Design review of the part built by this model. Coordinates are the model's own, in mm. A direction names the side the tool comes from. Round coordinates to 2 decimals unless told otherwise and drop trailing zeros. Loops run counter-clockwise (first coordinate to the right, second up) from the corner with the lowest first, then second, coordinate; pieces in that order, holes last. Notation, with made-up numbers: M -9.5,69.5 L 42.5,69.5 A21 ccw 42.5,77.5 Z; hole C 41.5,29.25 d8. An arc over 180 degrees is marked long. Use a Markdown table: item, result.
from build123d import *

# Parameters (mm, degrees)
SKETCH_W            = 120.815
SKETCH_H            = 65.873
PAD_DEPTH           = 25
POCKET_DEPTH        = 17
SKETCH002_R         = 0.8
HOLE_DEPTH          = 8.001
SKETCH003_W         = 10.80455
SKETCH003_H         = 10.011545
SKETCH003_W_2       = 3
SKETCH003_H_2       = 20
SKETCH003_W_3       = 21
SKETCH003_H_3       = 14
SKETCH003_W_4       = 17.5
SKETCH003_H_4       = 8
SKETCH003_W_5       = 4
SKETCH003_H_5       = 15
SKETCH003_W_6       = 39.832252
SKETCH003_H_6       = 6.416744
PAD001_DEPTH        = 14
HOLE001_D           = 3.5
HOLE001_DEPTH       = 20
HOLE001_CBORE_D     = 4.2
HOLE001_CBORE_DEPTH = 5
POCKET001_DEPTH     = 120.816


with BuildPart() as part:
    # Sketch → Pad (new body)
    with BuildSketch(Plane.XY):
        with Locations((50.4075, 22.9365)):
            Rectangle(SKETCH_W, SKETCH_H)
    extrude(amount=-PAD_DEPTH)

    # Sketch001 (on Face5 of Pad) → Pocket (cut)
    with BuildSketch(Plane.XY):
        Polygon((-0.5, 40.5), (-0.5, -0.5), (17.5, -0.5), (17.5, 5.25), (40.721178, 5.25), (40.721178, -0.5), (101.315, -0.5), (101.315, 40.5), (96.315, 40.5), (96.315, 50.5), (9.5, 50.5), (9.5, 40.5), align=None)
    extrude(amount=-POCKET_DEPTH, mode=Mode.SUBTRACT)

    # Sketch002 (on Face19 of Pocket) → Hole (cut, through all)
    with BuildSketch(Plane.XY.offset(-17)):
        with Locations((60.8, 35.99)):
            Circle(SKETCH002_R)
        with Locations((63.34, 35.99)):
            Circle(SKETCH002_R)
        with Locations((65.88, 35.99)):
            Circle(SKETCH002_R)
        with Locations((65.88, 33.45)):
            Circle(SKETCH002_R)
        with Locations((63.34, 33.45)):
            Circle(SKETCH002_R)
        with Locations((60.8, 33.45)):
            Circle(SKETCH002_R)
    extrude(amount=-HOLE_DEPTH, mode=Mode.SUBTRACT)

    # Sketch003 (on Face25 of Hole) → Pad001 (join)
    with BuildSketch(Plane.XY.offset(-17)):
        with Locations((82.816269, 15.264502)):
            Rectangle(SKETCH003_W, SKETCH003_H)
        with Locations((99.815, 30.5)):
            Rectangle(SKETCH003_W_2, SKETCH003_H_2)
        with Locations((51.221178, 6.5)):
            Rectangle(SKETCH003_W_3, SKETCH003_H_3)
        with Locations((8.75, 4)):
            Rectangle(SKETCH003_W_4, SKETCH003_H_4)
        with Locations((1.5, 33)):
            Rectangle(SKETCH003_W_5, SKETCH003_H_5)
        Polygon((58.883009, 23.721054), (58.883009, 29.721054), (68.383009, 29.721054), (68.383009, 50.5), (71.383009, 50.5), (71.383009, 23.721054), align=None)
        with Locations((34.88002, 25.574335)):
            Rectangle(SKETCH003_W_6, SKETCH003_H_6)
    extrude(amount=PAD001_DEPTH)

    # Hole001
    with Locations(Plane(origin=(0, 0, -25), x_dir=(1, 0, 0), z_dir=(0, 0, -1))):
        with Locations((-5.25, 5.25), (106.065, 5.25), (-5.25, -51.123), (106.065, -51.123)):
            CounterBoreHole(HOLE001_D / 2, HOLE001_CBORE_D / 2, HOLE001_CBORE_DEPTH, depth=HOLE001_DEPTH)

    # Sketch005 (on Face2 of Hole001) → Pocket001 (cut, through all)
    with BuildSketch(Plane(origin=(-10, 0, 0), x_dir=(0, -1, 0), z_dir=(-1, 0, 0))):
        Polygon((-55.873, -2), (-53.75168, -4.12132), (-55.873, -6.242641), align=None)
        Polygon((10, -2), (7.87868, -4.12132), (10, -6.242641), align=None)
    extrude(amount=-POCKET001_DEPTH, mode=Mode.SUBTRACT)


solid = part.part
1. Take a section at D-D on x = 89.5. Give the boundary of the cut face in (y, z), and give its area (3 significant figures).
Check values:
| item | result |
|---|---|
| outline | M -10,-25 L 55.87,-25 L 55.87,-6.24 L 53.75,-4.12 L 55.87,-2 L 55.87,0 L 50.5,0 L 50.5,-17 L -0.5,-17 L -0.5,0 L -10,0 L -10,-2 L -7.88,-4.12 L -10,-6.24 Z |
| area | 771 mm² |
2. Take a section at B-B on y = 42. Give the boundary of the cut face in (x, z) (3 decimals).
Check values:
| item | result |
|---|---|
| outline | M -10,-25 L 110.815,-25 L 110.815,0 L 96.315,0 L 96.315,-17 L 71.383,-17 L 71.383,-3 L 68.383,-3 L 68.383,-17 L 9.5,-17 L 9.5,0 L -10,0 Z |
3. Take a section at C-C on z = -12. Count the separate pieces of the cut face and the enclosed holes in it, and give its area (3 significant figures).
Check values:
| item | result |
|---|---|
| separate pieces | 3 |
| enclosed holes | 5 |
| area | 4,070 mm² |
4. Machinability: for faces 1 (the face through (-4.87, 52.83, -12.4)), 2 (the face through (69, 31, -3)), which of the approach directions +Z, -Z, +X, -X, +Y, -Y give a long, thin tool a straight path to every point of the face, cutting with its end or side? Answer none if there is none.
Check values:
| item | result |
|---|---|
| face 1 | -Z |
| face 2 | +Z |
5. Take a section at A-A on x = 53. Give the boundary of the cut face in (y, z).
Check values:
| item | result |
|---|---|
| outline | M -10,-25 L 55.87,-25 L 55.87,-6.24 L 53.75,-4.12 L 55.87,-2 L 55.87,0 L 50.5,0 L 50.5,-17 L 28.78,-17 L 28.78,-3 L 22.37,-3 L 22.37,-17 L 13.5,-17 L 13.5,-3 L -0.5,-3 L -0.5,0 L -10,0 L -10,-2 L -7.88,-4.12 L -10,-6.24 Z |
6. Insertion check: pin 1 (2 mm diameter, centred on x = 59, z = -6, fed in from +Y); pin 2 (5 mm diameter, centred on x = 81.5, y = 14, fed in from +Z); pin 3 (2 mm diameter, centred on x = 106.065, y = -5.25, fed in from -Z); pin 4 (1.8 mm diameter, centred on x = 63.34, y = 33.45, fed in from +Z). Each pin has a flat end and moves straight along its axis. Give the tip position at first contact, or say it passes through.
Check values:
| item | result |
|---|---|
| pin 1 | stops at y = 55.87 |
| pin 2 | stops at z = -3 |
| pin 3 | stops at z = -5 |
| pin 4 | stops at z = -17 |
7. Wall thickness on line 1 along Y through (x, z) = (65.88, -21.75); line 2 along X through (y, z) = (12, -14) (3 decimals); line 3 along X through (y, z) = (33.45, -19.75) (3 decimals): over which ranges is each line inside the solid? List them lowest first. Write a range as from..to.
Check values:
| item | result |
|---|---|
| line 1 | y = -10..32.65, 34.25..35.19, 36.79..55.87 |
| line 2 | x = -10..-0.5, 40.721..61.721, 77.414..88.219, 101.315..110.815 |
| line 3 | x = -10..60, 61.6..62.54, 64.14..65.08, 66.68..110.815 |
8. The part is to be moulded in two halves that separate along X. For faces 3 (the face through (110.815, 22, -12)), 4 (the face through (6, 40.5, -6)), say which applies: pulls with the +X half, pulls with the -X half, needs draft (parallel to the pull), parting line crosses it, or undercut.
Check values:
| item | result |
|---|---|
| face 3 | pulls with the +X half |
| face 4 | undercut |
